```python
from build123d import *

# Parameters (mm, degrees)
F0_W           = 127
F0_H           = 254
F1_DEPTH       = 254
F3_D           = 127
F3_CBORE_D     = 177.8
F3_CBORE_DEPTH = 127


with BuildPart() as f1:
    # F0 (on Top) → F1 (new body)
    with BuildSketch(Plane.XY):
        with Locations((63.5, 127)):
            Rectangle(F0_W, F0_H)
    extrude(amount=F1_DEPTH)

    # F3 (through all)
    with Locations(Plane(origin=(0, 0, 0), x_dir=(0, -1, 0), z_dir=(-1, 0, 0))):
        with Locations((-153.27017, 152.818576)):
            CounterBoreHole(F3_D / 2, F3_CBORE_D / 2, F3_CBORE_DEPTH)


solid = f1.part
```
Read the model definition and answer for the solid it produces. Units are mm, in the model's axes. Round coordinates to 2 decimals unless told otherwise and drop trailing zeros. Write each loop counter-clockwise with the first axis right and the second up, starting at its lowest first coordinate (ties: lowest second). Pieces come first, ordered by that corner, then holes. Notation, with made-up numbers: (17, 37.5) -> (60, 37.5) arc R24 cw to (60, 72.5) -> close; hole circle Ø10 at (57.5, 67). An arc over 180 degrees is marked (long way). Answer in a Markdown table with one row per item. Add a question column.
1) Determine the mould class of faces 1 (the face through (63, 129, 254)), 2 (the face through (62.611, 172.542, 66.033)), 3 (the face through (63, 0, 125)), 4 (the face through (63, 129, 0)) for opening direction Z: pulls with the +Z half, pulls with the -Z half, needs draft (parallel to the pull), parting line crosses it, or undercut.
2) Consider line 1 (Z direction, x = 110.5, y = 152); line 2 (Z direction, x = 9.5, y = 220.5); line 3 (Y direction, x = 52.5, z = 218.5). Determine where each line is inside the solid, lowest interval first.
3) Find section B-B, the plane z = 238. Determine the outline of the cut face in (x, y).
4) Given P1, Ø1.5, axis at y = 57, z = 117.5, coming from the -X side, flat-ended and moving along its own axis, determine where the tip first touches the part or whether it passes through.
5) Find section C-C, the plane x = 89. Determine the outline of the cut face in (y, z), and give its area (3 significant figures).
6) Find section A-A, the plane y = 218. Determine the outline of the cut face in (x, z), and give its area (3 significant figures).
Findings below:
| question | item | result |
|---|---|---|
| 1 | face 1 | pulls with the +Z half |
| 1 | face 2 | undercut |
| 1 | face 3 | needs draft |
| 1 | face 4 | pulls with the -Z half |
| 2 | line 1 | 0 to 63.93, 241.71 to 254 |
| 2 | line 2 | 0 to 94.65, 210.99 to 254 |
| 2 | line 3 | 0 to 93.36, 213.18 to 254 |
| 3 | outline | (0, 0) -> (127, 0) -> (127, 127.83) -> (0, 127.83) -> close; (0, 178.71) -> (127, 178.71) -> (127, 254) -> (0, 254) -> close |
| 4 | P1 | x = 0 |
| 5 | outline | (0, 0) -> (254, 0) -> (254, 254) -> (0, 254) -> close; hole circle Ø177.8 at (153.27, 152.82) |
| 5 | area | 39,700 mm² |
| 6 | outline | (0, 0) -> (127, 0) -> (127, 91.88) -> (0, 91.88) -> close; (0, 213.76) -> (127, 213.76) -> (127, 254) -> (0, 254) -> close |
| 6 | area | 16,800 mm² |
